Geometry: final body of the model. Coordinates: model frame, mm. Round coordinates to 2 decimals unless told otherwise and drop trailing zeros. Write each loop counter-clockwise with the first axis right and the second up, starting at its lowest first coordinate (ties: lowest second). Pieces come first, ordered by that corner, then holes. Notation, with made-up numbers: M -38.5,23 L 9.5,23 A18 ccw 9.5,28 Z; hole C 84,-12.5 d10. An arc over 180 degrees is marked long. Answer as CSV lines item,"result". Start each with the question number.
Q1. Section query B-B on x = -51.5. Output: boundary loops of the cut face in (y, z) (3 decimals), and give its area (3 significant figures).
Q2. Section query C-C on y = -1.75. Output: boundary loops of the cut face in (x, z).
Q3. Ray query, probe 1 along X at (y, z) = (-2.5, 38.1); probe 2 along X at (y, z) = (-1, -36). Return the intervals inside material, ascending.
Q4. Section query A-A on z = -38.1. Output: boundary loops of the cut face in (x, y) (3 decimals), and give its area (3 significant figures).
```python
from build123d import *

# Parameters (mm, degrees)
F0_W     = 203.2
F0_H     = 101.6
F1_DEPTH = 9.525
F2_D     = 11.1125
F2_DEPTH = 19.05
F2_TIP   = 3.3385318145


# Not quite as in the source:
# - a length typed as a fraction of an inch, garbled in the dataset ("3 / 203.2 mm" for 3/8 in), is restored


with BuildPart() as f1:
    # F0 (on Front) → F1 (new body)
    with BuildSketch(Plane.XZ):
        with Locations((1.4680749737, 0)):
            Rectangle(F0_W, F0_H)
    extrude(amount=F1_DEPTH)

    # F2
    with Locations(Plane(origin=(0, 0, 0), x_dir=(1, 0, 0), z_dir=(0, 1, 0))):
        with Locations((74.4930749737, -38.1), (-49.3319250263, 38.1), (-49.3319250263, -38.1), (74.4930749737, 38.1)):
            Hole(F2_D / 2, depth=F2_DEPTH)
            with Locations((0, 0, -(F2_DEPTH + F2_TIP / 2))):  # 118° drill point
                Cone(0, F2_D / 2, F2_TIP, mode=Mode.SUBTRACT)


solid = f1.part
```
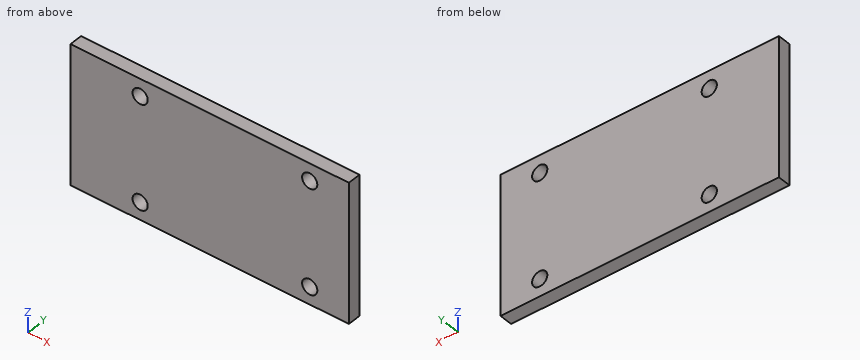
Entries:
1,outline,"M -9.525,-50.8 L 0,-50.8 L 0,-43.216 L -9.525,-43.216 Z; M -9.525,-32.984 L 0,-32.984 L 0,32.984 L -9.525,32.984 Z; M -9.525,43.216 L 0,43.216 L 0,50.8 L -9.525,50.8 Z"
1,area,"773 mm^2"
2,outline,"M -100.13,-50.8 L 103.07,-50.8 L 103.07,50.8 L -100.13,50.8 Z; hole C -49.33,-38.1 d11.11; hole C -49.33,38.1 d11.11; hole C 74.49,-38.1 d11.11; hole C 74.49,38.1 d11.11"
3,probe 1,"x = -100.13 to -54.89, -43.78 to 68.94, 80.05 to 103.07"
3,probe 2,"x = -100.13 to -54.48, -44.19 to 69.35, 79.64 to 103.07"
4,outline,"M -100.132,-9.525 L -54.888,-9.525 L -54.888,0 L -100.132,0 Z; M -43.776,-9.525 L 68.937,-9.525 L 68.937,0 L -43.776,0 Z; M 80.049,-9.525 L 103.068,-9.525 L 103.068,0 L 80.049,0 Z"
4,area,"1,720 mm^2"
